Could you check a few things on this drawing? It's one solid part, dimensions in mm from its lowest x, y, z. A direction names the side the tool comes from. Coordinates: 2 decimals unless noted, no trailing zeros. Order: outer loops, then holes, each group sorted by start corner. A loop starts at its lowest first (then second) coordinate and runs counter-clockwise, first axis right, second up.
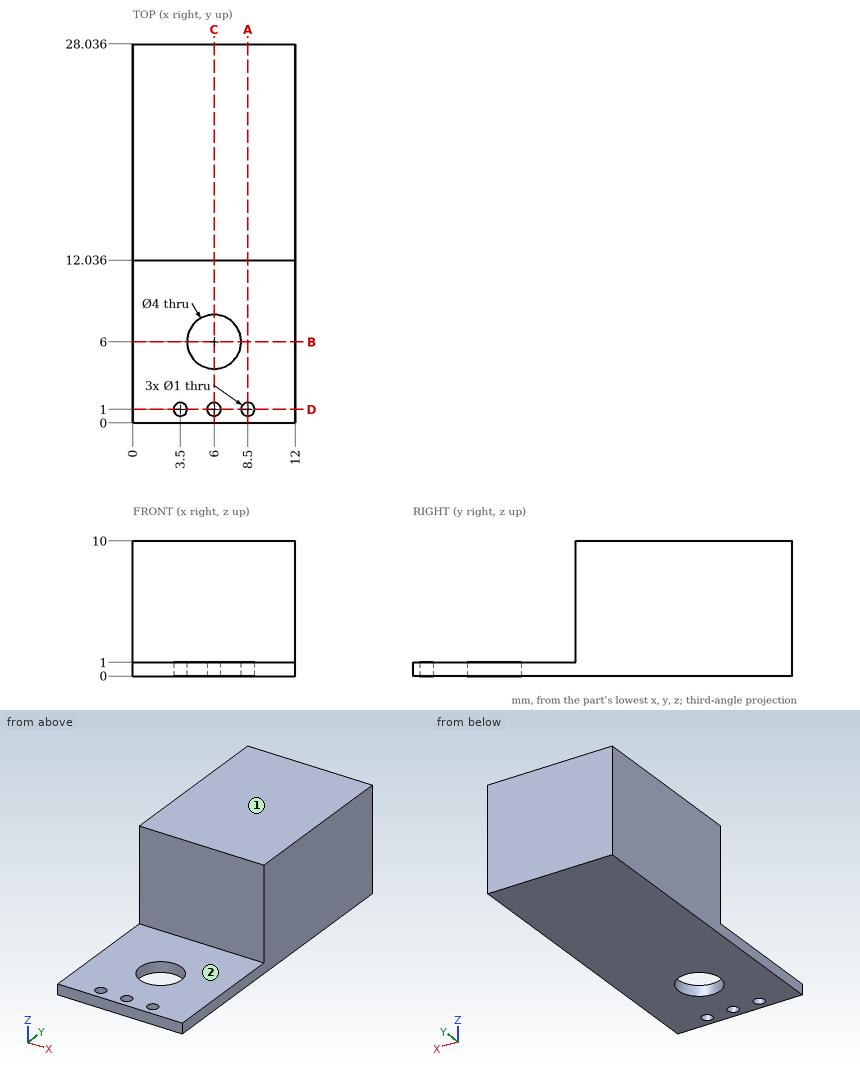
1. Please list where these lines run through material, in increasing order: probe 1 along Y at (x, z) = (8.5, 0.4); probe 2 along Y at (x, z) = (6, 0.6); probe 3 along Y at (x, z) = (1, 8.75).
Completed:
probe 1: y = 0 to 0.5, 1.5 to 28.04
probe 2: y = 0 to 0.5, 1.5 to 4, 8 to 28.04
probe 3: y = 12.04 to 28.04
2. I'm going to push flat-ended pins straight in: pin 1 (4.5 mm diameter, centred on x = 6.5, z = 7.5, fed in from -Y); pin 2 (5 mm diameter, centred on x = 6, y = 6, fed in from +Z). Where does each tip first touch, or does it pass through?
Completed:
pin 1: stops at y = 12.04
pin 2: stops at z = 1
3. Imagine slicing it at C-C on x = 6. Please give me the cut outline in (y, z).
Completed:
outline: (0, 0) - (0.5, 0) - (0.5, 1) - (0, 1) - close; (1.5, 0) - (4, 0) - (4, 1) - (1.5, 1) - close; (8, 0) - (28.04, 0) - (28.04, 10) - (12.04, 10) - (12.04, 1) - (8, 1) - close
4. On a 3-axis mill with a long thin cutter (end or side, diameter ignored), from which of +Z, -Z, +X, -X, +Y, -Y can I reach the whole of each face in a straight line? I mean the marked faces 1 and 2. Say none if no direction works.
Completed:
face 1: +Z, +X, -X, +Y, -Y
face 2: +Z, +X, -X, -Y
5. Imagine slicing it at A-A on x = 8.5. Please give me the cut outline in (y, z).
Completed:
outline: (0, 0) - (0.5, 0) - (0.5, 1) - (0, 1) - close; (1.5, 0) - (28.04, 0) - (28.04, 10) - (12.04, 10) - (12.04, 1) - (1.5, 1) - close
6. Imagine slicing it at B-B on y = 6. Please give me the cut outline in (x, z).
Completed:
outline: (0, 0) - (4, 0) - (4, 1) - (0, 1) - close; (8, 0) - (12, 0) - (12, 1) - (8, 1) - close
7. Imagine slicing it at D-D on y = 1. Please give me the cut outline in (x, z).
Completed:
outline: (0, 0) - (3, 0) - (3, 1) - (0, 1) - close; (4, 0) - (5.5, 0) - (5.5, 1) - (4, 1) - close; (6.5, 0) - (8, 0) - (8, 1) - (6.5, 1) - close; (9, 0) - (12, 0) - (12, 1) - (9, 1) - close
